Geometry: final body of the model. Coordinates: model frame, mm. Face numbers are marked on the shaded views. Give positions to 0.01 mm unless a question says otherwise; leave off trailing zeros. Order: outer loops, then holes, each group sorted by start corner. A loop starts at its lowest first (then second) coordinate and runs counter-clockwise, first axis right, second up. Notation, with made-up numbers: (57.25, 54) - (86.25, 54) arc R10 ccw to (86.25, 71) - close; hole circle Ø2 at (-7.5, 70). An arc over 180 degrees is marked (long way). One line per item, written item: value.
```python
from build123d import *

# Parameters (mm, degrees)
F3_R      = 5
F4_DEPTH  = 3
F8_DEPTH  = 3
F9_COUNT  = 29
F10_R     = 0.5
F11_DEPTH = 3


with BuildPart() as f4:
    # F3 (on Top) → F4 (new body)
    with BuildSketch(Plane.XY):
        Circle(F3_R)
    extrude(amount=F4_DEPTH)

    # F5 (on face) → F8 (join)
    with BuildSketch(Plane.XY.offset(3)):
        Polygon((5.2909918854, -0.2), (5.2909918854, 0.2), (4.9909918854, 0.3), (4.8909918854, 0.3), (4.8909918854, -0.3), (4.9909918854, -0.3), align=None)
    extrude(amount=-F8_DEPTH)

    # F9: F4 ×29 about axis
    f9_axis = Axis((0, 0, 0), (0, 0, -1))


with BuildPart() as f4_1:
    add(f4.part)
    for i in range(1, F9_COUNT):
        add(f4.part.rotate(f9_axis, i * 360 / F9_COUNT))

    # F10 (on face) → F11 (cut, through all)
    with BuildSketch(Plane(origin=(0, 0, 0), x_dir=(1, 0, 0), z_dir=(0, 0, -1))):
        Circle(F10_R)
    extrude(amount=-F11_DEPTH, mode=Mode.SUBTRACT)


solid = f4_1.part
```
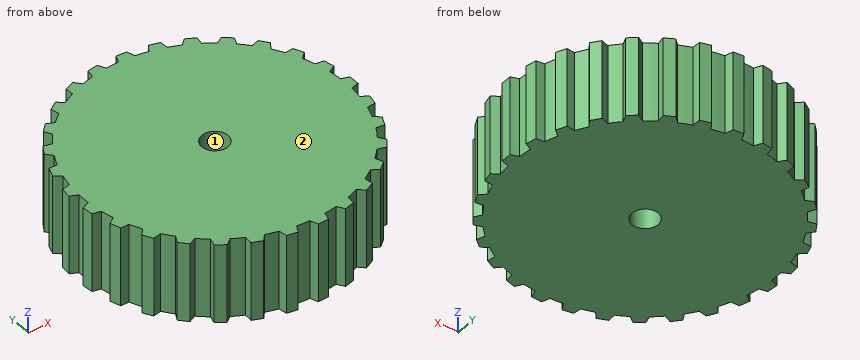
1) Section A-A, the plane y = 0. Return loops of the section in (x, z), then the cut area to 3 significant figures.
Answers below:
outline: (-5, 0) - (-0.5, 0) - (-0.5, 3) - (-5, 3) - close; (0.5, 0) - (5.29, 0) - (5.29, 3) - (0.5, 3) - close
area: 27.9 mm^2
2) Mould query, pull axis Y, two halves, no side actions, for the marked faces 1 and 2. Classes: released by +Y, released by -Y, zero draft, split by the parting line, or undercut.
Answers below:
face 1: undercut
face 2: zero draft
3) Material intervals for line 1 along Y through (x, z) = (-1.5, 0.4); line 2 along X through (y, z) = (-2, 0.9); line 3 along Y through (x, z) = (4, 2.15), sorted ascending.
Answers below:
line 1: -4.77 to 4.77
line 2: -4.58 to 4.84
line 3: -3.33 to 3.33
